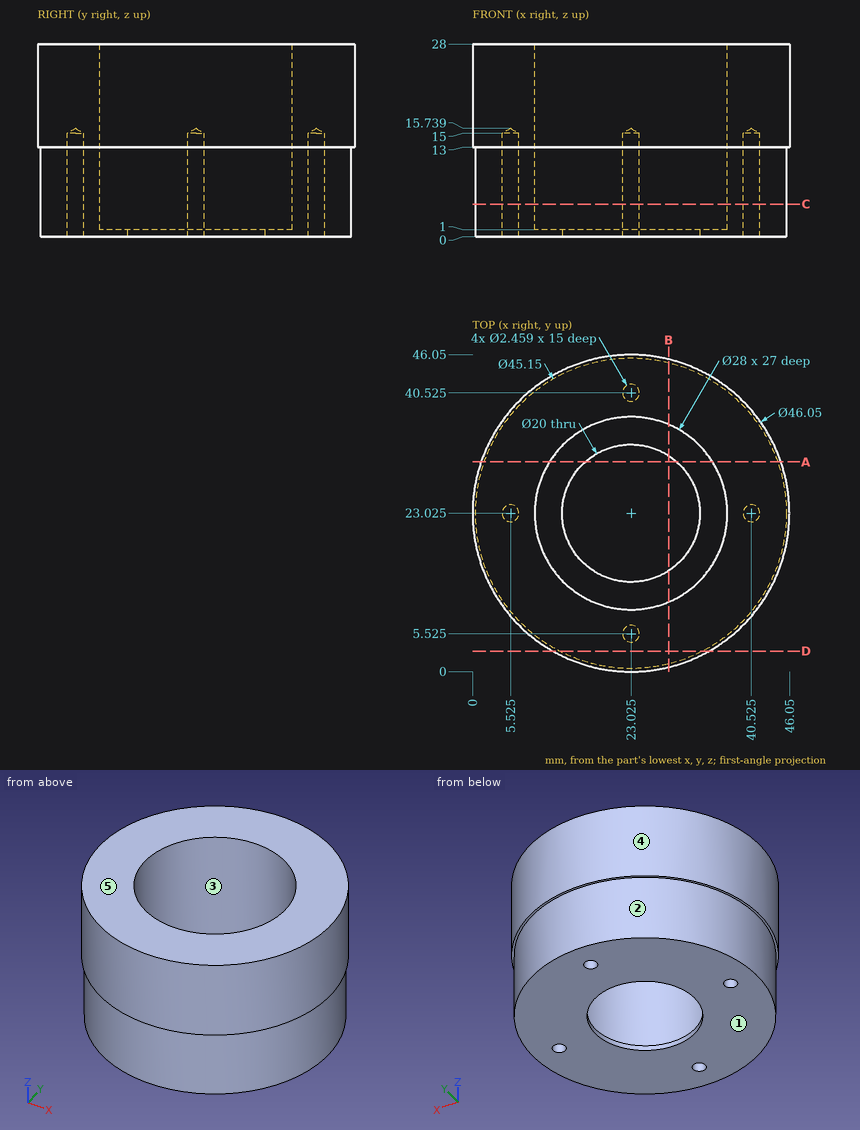
The figure shows three views and two pictorial views of one solid part (mm, origin at its lowest corner). Answer the questions. A direction names the side the tool comes from. Round coordinates to 2 decimals unless told otherwise and drop trailing zeros. Loops run counter-clockwise (first coordinate to the right, second up) from the corner with the lowest first, then second, coordinate; pieces in that order, holes last. Notation, with made-up numbers: (45, 35.5) - (65, 35.5) arc R20 ccw to (65, 48.5) - close; hole circle Ø11 at (-13, 16). An arc over 180 degrees is marked (long way). Use one line per item in the form item = value. Start each with the question number.
(1) Which of the six approach directions +Z, -Z, +X, -X, +Y, -Y give full straight-line access (tool end or side, diameter ignored) to the marked faces 1 and 2?
(2) Consider line 1 (X direction, y = 22, z = 8.25) (1 decimal); line 2 (X direction, y = 17.5, z = 3.25); line 3 (X direction, y = 41, z = 5.5). Determine where each line is inside the solid, lowest interval first.
(3) Flat-ended cylindrical pins translate along their axes: P1, Ø8, axis at x = 27.5, z = 17, coming from the -Y side (3 decimals); P2, Ø5, axis at x = 6.5, z = 14, coming from the -Y side (1 decimal); P3, Ø6, axis at x = 15, z = 25, coming from the +Y side (3 decimals). Find the tip coordinate at first contact, or state that the pin passes through.
(4) Determine the mould class of the marked faces 3, 4 and 5 for opening direction X: +X half, -X half, draft (parallel to the pull), parting line (faces both ways), or undercut.
(5) Find section A-A on y = 30.5. Determine the outline of the cut face in (x, z).
(6) Find section D-D on y = 3. Determine the outline of the cut face in (x, z).
(7) Find section B-B on x = 28.5. Determine the outline of the cut face in (y, z), and give its area (3 significant figures).
(8) Find section C-C on z = 4.75. Give the number of separate pieces and of enclosed holes in the cut face, and give its area (3 significant figures).
Answer list:
q1.face_1 = -Z, +X, -X, +Y, -Y
q1.face_2 = -Z
q2.line_1 = 0.5 to 4.8, 6.2 to 9.1, 37 to 39.8, 41.2 to 45.6
q2.line_2 = 1.14 to 10.16, 35.89 to 44.91
q2.line_3 = 9.37 to 21.89, 24.16 to 36.68
q3.P1 = 0.005
q3.P2 = 4.8
q3.P3 = 45.495
q4.face_3 = undercut
q4.face_4 = parting line
q4.face_5 = draft
q5.outline = (1.25, 13) - (1.72, 13) - (1.72, 0) - (16.38, 0) - (16.38, 1) - (11.19, 1) - (11.19, 28) - (1.25, 28) - close; (29.67, 0) - (44.33, 0) - (44.33, 13) - (44.8, 13) - (44.8, 28) - (34.86, 28) - (34.86, 1) - (29.67, 1) - close
q6.outline = (11.66, 13) - (12.6, 13) - (12.6, 0) - (33.45, 0) - (33.45, 13) - (34.39, 13) - (34.39, 28) - (11.66, 28) - close
q7.outline = (0.66, 13) - (1.12, 13) - (1.12, 0) - (14.66, 0) - (14.66, 1) - (10.14, 1) - (10.14, 28) - (0.66, 28) - close; (31.39, 0) - (44.93, 0) - (44.93, 13) - (45.39, 13) - (45.39, 28) - (35.91, 28) - (35.91, 1) - (31.39, 1) - close
q7.area = 528 mm^2
q8.separate_pieces = 1
q8.enclosed_holes = 5
q8.area = 966 mm^2
